Source: CAD feature listing. Evaluate the final solid. Frame: model axes, mm. Coordinates: 2 decimals unless noted, no trailing zeros. Loops run counter-clockwise (first coordinate to the right, second up) from the corner with the lowest first, then second, coordinate; pieces in that order, holes last. Notation, with made-up numbers: (51.25, -33.5) -> (85.25, -33.5) arc R33 ccw to (85.25, -2.5) -> close; hole circle Ø5 at (-27, -17.5). An arc over 180 degrees is marked (long way). One line per question, with ' | ' between items. Start each with the question number.
```python
from build123d import *

# Parameters (mm, degrees)
SKETCH2_W           = 23.74600026
SKETCH2_H           = 9.873000066
BOSS_EXTRUDE1_DEPTH = 8.3185
SKETCH3_R           = 2.99974
CUT_EXTRUDE1_DEPTH  = 18.539717918
SKETCH4_R           = 0.254
CUT_EXTRUDE2_DEPTH  = 2.54


with BuildPart() as part:
    # Sketch2 → Boss-Extrude1 (new body)
    with BuildSketch(Plane(origin=(0, 0, 0), x_dir=(1, 0, 0), z_dir=(0, 1, 0))):
        Rectangle(SKETCH2_W, SKETCH2_H)
    extrude(amount=BOSS_EXTRUDE1_DEPTH)

    # Sketch3 → Cut-Extrude1 (cut, through all)
    with BuildSketch(Plane.XY.offset(4.936500033)):
        with Locations((0, 8.3185)):
            Circle(SKETCH3_R)
    extrude(amount=-CUT_EXTRUDE1_DEPTH, mode=Mode.SUBTRACT)

    # Sketch4 → Cut-Extrude2 (cut)
    with BuildSketch(Plane(origin=(0, 8.3185, 0), x_dir=(1, 0, 0), z_dir=(0, 1, 0))):
        with Locations(Location((-6.99999997, 0, 0), (0, 0, 270))):
            Circle(SKETCH4_R)
        with Locations(Location((6.99999997, 0, 0), (0, 0, 90))):
            Circle(SKETCH4_R)
    extrude(amount=-CUT_EXTRUDE2_DEPTH, mode=Mode.SUBTRACT)


solid = part.part
```
(1) Cut plane B-B, the plane x = 7. Return the cut outline in (y, z), and give its area (3 significant figures).
(2) Ray query, L1, parallel to Z at x = 7, y = 7.3; L2, parallel to X at y = 7.6, z = 0; L3, parallel to X at y = 6.4, z = 0. Return the intervals inside material, ascending.
(3) Cut plane D-D, the plane z = 3. Return the cut outline in (x, y), and give its area (3 significant figures).
(4) Draft query along X for faces 1 (the flat face through (-11.873, 4, 0)), 2 (the cylindrical face through (-0.07, 5.32, 0.07)), 3 (the flat face through (7.4, 8.318, -0.1)). Return one class per face: pulls with the +X half, pulls with the -X half, needs draft (parallel to the pull), parting line crosses it, or undercut.
(5) Cut plane A-A, the plane y = 6.5. Return the cut outline in (x, z), and give its area (3 significant figures).
(6) Cut plane C-C, the plane z = 0. Return the cut outline in (x, y).
Here are the results:
1) outline: (0, -4.94) -> (8.32, -4.94) -> (8.32, -0.25) -> (5.78, -0.25) -> (5.78, 0.25) -> (8.32, 0.25) -> (8.32, 4.94) -> (0, 4.94) -> close | area: 80.8 mm2
2) L1: z = -4.94 to -0.25, 0.25 to 4.94 | L2: x = -11.87 to -7.25, -6.75 to -2.91, 2.91 to 6.75, 7.25 to 11.87 | L3: x = -11.87 to -7.25, -6.75 to -2.31, 2.31 to 6.75, 7.25 to 11.87
3) outline: (-11.87, 0) -> (11.87, 0) -> (11.87, 8.32) -> (3, 8.32) arc R3 cw to (-3, 8.32) -> (-11.87, 8.32) -> close | area: 183 mm2
4) face 1: pulls with the -X half | face 2: undercut | face 3: needs draft
5) outline: (-11.87, -4.94) -> (-2.39, -4.94) -> (-2.39, 4.94) -> (-11.87, 4.94) -> close; (2.39, -4.94) -> (11.87, -4.94) -> (11.87, 4.94) -> (2.39, 4.94) -> close; hole circle Ø0.51 at (-7, 0); hole circle Ø0.51 at (7, 0) | area: 187 mm2
6) outline: (-11.87, 0) -> (11.87, 0) -> (11.87, 8.32) -> (7.25, 8.32) -> (7.25, 5.78) -> (6.75, 5.78) -> (6.75, 8.32) -> (3, 8.32) arc R3 cw to (-3, 8.32) -> (-6.75, 8.32) -> (-6.75, 5.78) -> (-7.25, 5.78) -> (-7.25, 8.32) -> (-11.87, 8.32) -> close
